Design review of the part built by this model. Coordinates are the model's own, in mm. Coordinates: 2 decimals unless noted, no trailing zeros. Write each loop counter-clockwise with the first axis right and the second up, starting at its lowest first coordinate (ties: lowest second). Pieces come first, ordered by that corner, then holes.
```python
from build123d import *

# Parameters (mm, degrees)
ESQUISSE1_R             = 0.625
BOSS_EXTRU_1_DEPTH      = 11.662554
BOSS_EXTRU_1_DEPTH_BACK = 11.662554
ESQUISSE2_R             = 0.33
BOSS_EXTRU_2_DEPTH      = 1.837446
ESQUISSE3_R             = 0.33
BOSS_EXTRU_3_DEPTH      = 1.837446
D_ME1_FACE_RADIUS       = 0.33
D_ME1_HEIGHT            = 0.25
D_ME2_FACE_RADIUS       = 0.33
D_ME2_HEIGHT            = 0.25
CONG_1_R                = 0.15


with BuildPart() as part:
    # Esquisse1 → Boss.-Extru.1 (new body, two sides)
    with BuildSketch(Plane.XY) as boss_extru_1_sk:
        Circle(ESQUISSE1_R)
    extrude(amount=BOSS_EXTRU_1_DEPTH)
    extrude(boss_extru_1_sk.sketch, amount=-BOSS_EXTRU_1_DEPTH_BACK)

    # Esquisse2 → Boss.-Extru.2 (add)
    with BuildSketch(Plane.XY.offset(11.662554)):
        Circle(ESQUISSE2_R)
    extrude(amount=BOSS_EXTRU_2_DEPTH)

    # Esquisse3 → Boss.-Extru.3 (add)
    with BuildSketch(Plane(origin=(0, 0, -11.662554), x_dir=(-1, 0, 0), z_dir=(0, 0, -1))):
        Circle(ESQUISSE3_R)
    extrude(amount=BOSS_EXTRU_3_DEPTH)

    # D_me1: a dome of height H over a round flat face of radius A is a cap of a sphere of radius (A * A + H * H) / (2 * H)
    d_me1_r = (D_ME1_FACE_RADIUS * D_ME1_FACE_RADIUS + D_ME1_HEIGHT * D_ME1_HEIGHT) / (2 * D_ME1_HEIGHT)
    d_me1_base = Plane((0, 0, 13.5), z_dir=(0, 0, 1))
    with Locations(d_me1_base.offset(D_ME1_HEIGHT - d_me1_r)):
        d_me1_ball = Sphere(d_me1_r, mode=Mode.PRIVATE)
    add(split(d_me1_ball, bisect_by=d_me1_base, keep=Keep.TOP, mode=Mode.PRIVATE))

    # D_me2: a dome of height H over a round flat face of radius A is a cap of a sphere of radius (A * A + H * H) / (2 * H)
    d_me2_r = (D_ME2_FACE_RADIUS * D_ME2_FACE_RADIUS + D_ME2_HEIGHT * D_ME2_HEIGHT) / (2 * D_ME2_HEIGHT)
    d_me2_base = Plane((0, 0, -13.5), z_dir=(0, 0, -1))
    with Locations(d_me2_base.offset(D_ME2_HEIGHT - d_me2_r)):
        d_me2_ball = Sphere(d_me2_r, mode=Mode.PRIVATE)
    add(split(d_me2_ball, bisect_by=d_me2_base, keep=Keep.TOP, mode=Mode.PRIVATE))

    # Cong_1
    cong_1_edges = [part.edges().sort_by_distance(p)[0] for p in [
        (-0.625, 0, -11.662554),
        (-0.625, 0, 11.662554),
    ]]
    fillet(cong_1_edges, radius=CONG_1_R)


solid = part.part
```
(1) Consider section A-A (x = 0). Give the boundary of the cut face in (y, z) (3 decimals).
(2) Consider section C-C (z = -10). Give the boundary of the cut face in (x, y) (3 decimals), plus the area to 3 significant figures.
(3) Wall thickness on line 1 (Z direction, x = 0, y = 0.45); line 2 (Y direction, x = -0.05, z = -6.75); line 3 (X direction, y = -0.4, z = 2.25): over which ranges is each line inside the solid? List them lowest first.
Results:
1. outline: (-0.625, -11.513) arc R0.15 ccw to (-0.475, -11.663) - (-0.33, -11.663) - (-0.33, -13.5) arc R0.343 ccw to (0.33, -13.5) - (0.33, -11.663) - (0.475, -11.663) arc R0.15 ccw to (0.625, -11.513) - (0.625, 11.513) arc R0.15 ccw to (0.475, 11.663) - (0.33, 11.663) - (0.33, 13.5) arc R0.343 ccw to (-0.33, 13.5) - (-0.33, 11.663) - (-0.475, 11.663) arc R0.15 ccw to (-0.625, 11.513) - close
2. outline: circle Ø1.25 at (0, 0)
2. area: 1.23 mm2
3. line 1: z = -11.66 to 11.66
3. line 2: y = -0.62 to 0.62
3. line 3: x = -0.48 to 0.48
